Autodesk Fusion 360 part; units mm, degrees
sketch "スケッチ1" plane through (0, 0, 0) normal (1, 0, 0) x (0, 1, 0)
  line L0 (-40, 36.5) -> (40, 36.5)
  line L1 (40, 36.5) -> (40, -13.5)
  line L2 (20, -33.5) -> (-20, -33.5)
  line L3 (-40, -13.5) -> (-40, 36.5)
  arc A0 (20, -33.5) -> (40, -13.5) centre (20, -13.5) ccw
  arc A1 (-40, -13.5) -> (-20, -33.5) centre (-20, -13.5) ccw
  line L4 (-42, 38.5) -> (42, 38.5)
  line L5 (42, 38.5) -> (42, -13.5)
  line L6 (20, -35.5) -> (-20, -35.5)
  line L7 (-42, -13.5) -> (-42, 38.5)
  arc A2 (20, -35.5) -> (42, -13.5) centre (20, -13.5) ccw
  arc A3 (-42, -13.5) -> (-20, -35.5) centre (-20, -13.5) ccw
  point P0 (-40, -33.5)
  dimension "d1" = 80
  dimension "d2" = 70
  dimension "d3" = 33.5
  dimension "d4" = 40
  dimension "d5" = 20
  dimension "d6" = 20
  dimension "d7" = 2
  dimension "d8" = 2
  dimension "d9" = 2
  dimension "d10" = 2
  dimension "d11" = 22
  dimension "d12" = 22
extrude "押し出し1" add sketch "スケッチ1" along normal mid plane 176.6
sketch "スケッチ2" plane through (0, 0, 0) normal (0, 0, 1) x (1, 0, 0)
  line L0 (-90, 35) -> (90, 35)
  line L1 (90, 35) -> (90, -35)
  line L2 (90, -35) -> (-90, -35)
  line L3 (-90, -35) -> (-90, 35)
  dimension "d15" = 180
  dimension "d16" = 90
  dimension "d17" = 70
  dimension "d18" = 35
extrude "押し出し2" cut sketch "スケッチ2" along normal blind 50
sketch "スケッチ3" plane through (0, 0, 0) normal (0, 1, 0) x (1, 0, 0)
  line L0 (74.5, -45.5) -> (-74.5, -45.5)
  line L1 (-74.5, -45.5) -> (-74.5, 4.5)
  line L2 (-74.5, 4.5) -> (74.5, 4.5)
  line L3 (74.5, 4.5) -> (74.5, -45.5)
  dimension "d21" = 149
  dimension "d22" = 74.5
  dimension "d23" = 50
  dimension "d29" = 4.5
extrude "押し出し3" cut sketch "スケッチ3" along normal blind 45
fillet "フィレット1" radius 5 2 edges at (74.5, 41, -4.5) (-74.5, 41, -4.5)
equation "d3 = ( 67 / 2 ) * 1 mm"
equation "d4 = ( 80 / 2 ) * 1 mm"
equation "d13 = ( 176.6 / 2 ) * 1 mm"
equation "d17 = 80 mm - 10 mm"
equation "d18 = ( 70 / 2 ) * 1 mm"
equation "d22 = ( 149 / 2 ) * 1 mm"
The model under review builds one solid part; all positions refer to its coordinate system, in mm. A direction names the side the tool comes from. Coordinates: 2 decimals unless noted, no trailing zeros. Write each loop counter-clockwise with the first axis right and the second up, starting at its lowest first coordinate (ties: lowest second). Pieces come first, ordered by that corner, then holes. Notation, with made-up numbers: (20, 30) - (72, 30) arc R10 ccw to (72, 49) - close; hole circle Ø3 at (63.5, 45). An arc over 180 degrees is marked (long way). Answer in a Markdown table with one row per item. Add a question column.
Q1. Draft analysis for pull direction X (two halves, no side actions). For faces 6 (the face through (-88.3, 0, -34)), 7 (the face through (-1, -42, 12)), 8 (the face through (74.5, 40.3, 20.8)), state which applies: +X half, -X half, draft (parallel to the pull), parting line (faces both ways), or undercut.
Q2. Consider section D-D on y = -14.5. Give the boundary of the cut face in (x, z), then the cut area to 3 significant figures.
Q3. Consider section B-B on z = 27. Give the boundary of the cut face in (x, y), then the cut area to 3 significant figures.
Q4. Consider section C-C on x = 4. Give the boundary of the cut face in (y, z).
Q5. Clearance check with flat-ended pins moving along their axes: pin 1 (3 mm diameter, centred on x = -51.5, y = -32.5, fed in from -Z); pin 2 (1 mm diameter, centred on x = 68.5, z = -22.5, fed in from +Y); pin 3 (1.5 mm diameter, centred on x = 51.5, y = -22.5, fed in from +Z). State where each tip first meets the part, or that it passes through.
Q6. Consider section A-A on z = -10. Give the boundary of the cut face in (x, y).
Q7. For faces 1 (the face through (-1, -38, 36.5)), 2 (the face through (-1, 0, -33.5)), 3 (the face through (73.07, 41.01, -3)), 4 (the face through (-1.24, -35.38, -29.23)), 5 (the face through (-81, 38, 38.5)), list the 3-axis set-ups (+Z, -Z, +X, -X, +Y, -Y) from which the entire face can be reached by the end or side of a thin tool; tool diameter is ignored.
Q8. To check wall thickness, follow line 1 along Z through (x, y) = (46, 19.5); line 2 along Y through (x, z) = (77.5, 4); line 3 along Y through (x, z) = (66, 31). State the ranges of each line that lie inside material, in increasing order. Write a range as from..to.
Answers below:
| question | item | result |
|---|---|---|
| 1 | face 6 | -X half |
| 1 | face 7 | draft |
| 1 | face 8 | undercut |
| 2 | outline | (-88.3, -35.5) - (88.3, -35.5) - (88.3, -33.5) - (-88.3, -33.5) - close |
| 2 | area | 353 mm² |
| 3 | outline | (-88.3, -42) - (88.3, -42) - (88.3, -40) - (-88.3, -40) - close; (-88.3, 40) - (-74.5, 40) - (-74.5, 42) - (-88.3, 42) - close; (74.5, 40) - (88.3, 40) - (88.3, 42) - (74.5, 42) - close |
| 3 | area | 408 mm² |
| 4 | outline | (-42, -13.5) arc R22 ccw to (-20, -35.5) - (20, -35.5) arc R22 ccw to (42, -13.5) - (42, -4.5) - (40, -4.5) - (40, -13.5) arc R20 cw to (20, -33.5) - (-20, -33.5) arc R20 cw to (-40, -13.5) - (-40, 36.5) - (-35, 36.5) - (-35, 38.5) - (-42, 38.5) - close |
| 5 | pin 1 | z = -32.55 |
| 5 | pin 2 | y = 40.29 |
| 5 | pin 3 | z = -33.23 |
| 6 | outline | (-88.3, -42) - (88.3, -42) - (88.3, -40) - (-88.3, -40) - close; (-88.3, 40) - (88.3, 40) - (88.3, 42) - (-88.3, 42) - close |
| 7 | face 1 | +X, -X |
| 7 | face 2 | +Z, +X, -X |
| 7 | face 3 | +Z, +Y |
| 7 | face 4 | -Z, +X, -X, -Y |
| 7 | face 5 | +Z, +X, -X, +Y, -Y |
| 8 | line 1 | -35.5..-33.5 |
| 8 | line 2 | -42..-40, 40..42 |
| 8 | line 3 | -42..-40 |
